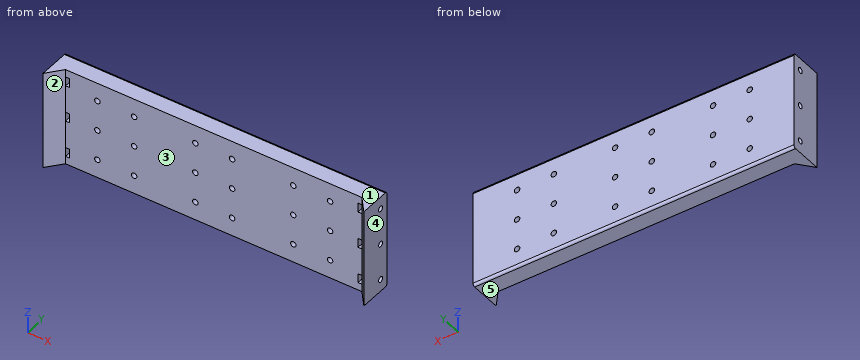
from build123d import *

# Parameters (mm, degrees)
SKETCH1_W           = 262
SKETCH1_H           = 80
BOSS_EXTRUDE1_DEPTH = 15
SKETCH2_R           = 2.25
CUT_EXTRUDE1_DEPTH  = 40
CUT_EXTRUDE2_DEPTH  = 3.2
SKETCH4_R           = 2.25
CUT_EXTRUDE3_DEPTH  = 138.789694825
LPATTERN1_COUNT     = 2
LPATTERN1_PITCH     = 80
LPATTERN1_COL_COUNT = 2
LPATTERN1_COL_PITCH = 80
FILLET1_R           = 2
BOSS_EXTRUDE2_DEPTH = 80


with BuildPart() as part:
    # Sketch1 → Boss-Extrude1 (new body)
    with BuildSketch(Plane(origin=(0, 0, 0), x_dir=(1, 0, 0), z_dir=(0, 1, 0))):
        Rectangle(SKETCH1_W, SKETCH1_H)
    extrude(amount=BOSS_EXTRUDE1_DEPTH)

    # Sketch2 → Cut-Extrude1 (cut)
    with BuildSketch(Plane.ZY.offset(131)):
        with Locations((0, 7.5)):
            Circle(SKETCH2_R)
        with Locations((-30, 7.5)):
            Circle(SKETCH2_R)
        with Locations(Location((30, 7.5, 0), (0, 0, 180))):
            Circle(SKETCH2_R)
    cut_extrude1 = extrude(amount=-CUT_EXTRUDE1_DEPTH, mode=Mode.SUBTRACT)

    # Sketch3 → Cut-Extrude2 (cut)
    with BuildSketch(Plane.ZY.offset(121)):
        Polygon((-33.75, 5.334936491), (-33.75, 0), (-26.25, 0), (-26.25, 5.334936491), (-26.25, 9.665063509), (-30, 11.830127019), (-33.75, 9.665063509), align=None)
        Polygon((0, 11.830127019), (-3.75, 9.665063509), (-3.75, 5.334936491), (-3.75, 0), (3.75, 0), (3.75, 5.334936491), (3.75, 9.665063509), align=None)
        Polygon((33.75, 5.334936491), (33.75, 0), (26.25, 0), (26.25, 5.334936491), (26.25, 9.665063509), (30, 11.830127019), (33.75, 9.665063509), align=None)
    cut_extrude2 = extrude(amount=-CUT_EXTRUDE2_DEPTH, mode=Mode.SUBTRACT)

    # Mirror1: Cut-Extrude1, Cut-Extrude2 across plane
    add(cut_extrude1.mirror(Plane(origin=(0, 0, 0), x_dir=(0, 0, 1), z_dir=(1, 0, 0))), mode=Mode.SUBTRACT)
    add(cut_extrude2.mirror(Plane(origin=(0, 0, 0), x_dir=(0, 0, 1), z_dir=(1, 0, 0))), mode=Mode.SUBTRACT)

    # Sketch4 → Cut-Extrude3 (cut, through all)
    with BuildSketch(Plane(origin=(0, 15, 0), x_dir=(1, 0, 0), z_dir=(0, 1, 0))):
        with Locations(Location((-15, 0, 0), (0, 0, 270))):
            Circle(SKETCH4_R)
        with Locations(Location((-15, 25, 0), (0, 0, 270))):
            Circle(SKETCH4_R)
        with Locations(Location((-15, -25, 0), (0, 0, 90))):
            Circle(SKETCH4_R)
        with Locations(Location((15, -25, 0), (0, 0, 270))):
            Circle(SKETCH4_R)
        with Locations(Location((15, 0, 0), (0, 0, 90))):
            Circle(SKETCH4_R)
        with Locations(Location((15, 25, 0), (0, 0, 90))):
            Circle(SKETCH4_R)
    cut_extrude3 = extrude(amount=-CUT_EXTRUDE3_DEPTH, mode=Mode.SUBTRACT)

    # LPattern1: Cut-Extrude3 ×2
    with Locations(*[(i * LPATTERN1_PITCH, 0, 0) for i in range(1, LPATTERN1_COUNT)]):
        add(cut_extrude3, mode=Mode.SUBTRACT)

    # LPattern1 col: Cut-Extrude3 ×2
    with Locations(*[(-i * LPATTERN1_COL_PITCH, 0, 0) for i in range(1, LPATTERN1_COL_COUNT)]):
        add(cut_extrude3, mode=Mode.SUBTRACT)

    # Fillet1
    fillet1_edges = [part.edges().sort_by_distance(p)[0] for p in [
        (0, 15, 40),
        (0, 15, -40),
    ]]
    fillet(fillet1_edges, radius=FILLET1_R)

    # Sketch7 → Boss-Extrude2 (add, through all)
    with BuildSketch(Plane.XY.offset(40)):
        Polygon((-131, 0), (-131, -12), (-121, 0), align=None)
    boss_extrude2 = extrude(amount=-BOSS_EXTRUDE2_DEPTH)

    # Mirror2: Boss-Extrude2 across plane
    add(boss_extrude2.mirror(Plane(origin=(0, 0, 0), x_dir=(0, 0, 1), z_dir=(1, 0, 0))))


solid = part.part
Input: part model. Units: mm. Frame: model coordinates. Face numbers are marked on the shaded views. A direction names the side the tool comes from. Coordinates: 2 decimals unless noted, no trailing zeros. Loops run counter-clockwise (first coordinate to the right, second up) from the corner with the lowest first, then second, coordinate; pieces in that order, holes last. Notation, with made-up numbers: (-32.75, -1.5) -> (-2.75, -1.5) arc R27 cw to (-2.75, 22.5) -> close; hole circle Ø4 at (17.5, -39.5). An arc over 180 degrees is marked (long way). One line per item, written item: value.
(1) Draft query along X for the marked faces 3, 4 and 5. Return one class per face: pulls with the +X half, pulls with the -X half, needs draft (parallel to the pull), parting line crosses it, or undercut.
Answer below:
face 3: undercut
face 4: pulls with the +X half
face 5: needs draft
(2) Set-up query: the marked faces 1 and 2. Return all of +Z, -Z, +X, -X, +Y, -Y with unobstructed straight access to the full face (end or side cutting, diameter ignored); none if empty.
Answer below:
face 1: +Z, +X, -X, +Y, -Y
face 2: +Z, -Z, -Y
(3) Cut plane D-D (z = 19.5). Output: boundary loops of the cut face in (x, y).
Answer below:
outline: (-131, -12) -> (-121, 0) -> (121, 0) -> (131, -12) -> (131, 15) -> (-131, 15) -> close
(4) Pin query (flat end, axial travel): pin 1 Ø6 at (y, z) = (7.5, 0) entering from -X; pin 2 Ø3.5 at (y, z) = (7.5, -30) entering from -X; pin 3 Ø10 at (x, z) = (37.5, -13) entering from -Y; pin 4 Ø4 at (x, z) = (95, 25) entering from +Y. Return the tip coordinate at first contact, or that it passes through.
Answer below:
pin 1: stops at x = -131
pin 2: stops at x = -91
pin 3: stops at y = 0
pin 4: passes through
(5) Cut plane B-B (y = -3.5). Output: boundary loops of the cut face in (x, z).
Answer below:
outline: (-131, -40) -> (-123.92, -40) -> (-123.92, 40) -> (-131, 40) -> close; (123.92, -40) -> (131, -40) -> (131, 40) -> (123.92, 40) -> close
(6) Cut plane C-C (x = 65). Output: boundary loops of the cut face in (y, z).
Answer below:
outline: (0, -40) -> (13, -40) arc R2 ccw to (15, -38) -> (15, -27.25) -> (0, -27.25) -> close; (0, -22.75) -> (15, -22.75) -> (15, -2.25) -> (0, -2.25) -> close; (0, 2.25) -> (15, 2.25) -> (15, 22.75) -> (0, 22.75) -> close; (0, 27.25) -> (15, 27.25) -> (15, 38) arc R2 ccw to (13, 40) -> (0, 40) -> close
(7) Ray query, line 1 along Z through (x, y) = (120, 2); line 2 along Z through (x, y) = (128, 7.5); line 3 along Y through (x, z) = (-111, 0). Return the intervals inside material, ascending.
Answer below:
line 1: z = -40 to -33.75, -26.25 to -3.75, 3.75 to 26.25, 33.75 to 40
line 2: z = -40 to -32.25, -27.75 to -2.25, 2.25 to 27.75, 32.25 to 40
line 3: y = 0 to 5.25, 9.75 to 15
(8) Cut plane A-A (x = -112). Output: boundary loops of the cut face in (y, z).
Answer below:
outline: (0, -40) -> (13, -40) arc R2 ccw to (15, -38) -> (15, 38) arc R2 ccw to (13, 40) -> (0, 40) -> close; hole circle Ø4.5 at (7.5, -30); hole circle Ø4.5 at (7.5, 0); hole circle Ø4.5 at (7.5, 30)
